The model under review builds one solid part; all positions refer to its coordinate system, in mm. Face numbers are marked on the shaded views. A direction names the side the tool comes from. Give positions to 0.01 mm unless a question says otherwise; leave off trailing zeros. Order: outer loops, then holes, each group sorted by start corner. A loop starts at its lowest first (then second) coordinate and runs counter-clockwise, first axis right, second up. Notation, with made-up numbers: (-3.75, 4) -> (50.25, 4) arc R22 cw to (50.25, 29) -> close; hole circle Ø9 at (63.5, 55). An arc over 180 degrees is marked (long way). Use one line per item in the form item = value.
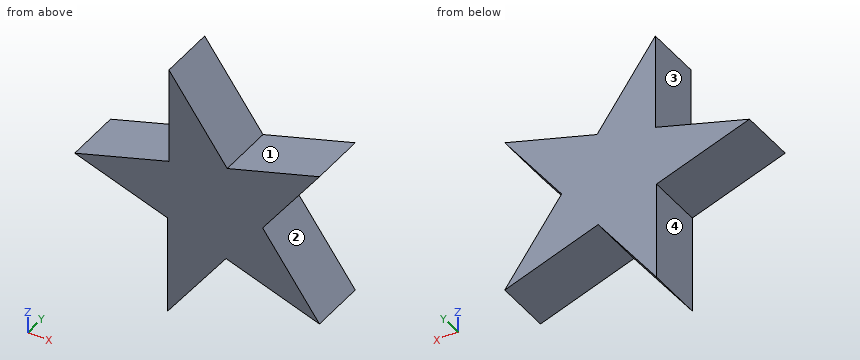
Autodesk Inventor part; units mm, degrees
ref_plane "YZ Plane" through (0, 0, 0) normal (1, 0, 0) x (0, 1, 0)
ref_plane "XZ Plane" through (0, 0, 0) normal (0, 1, 0) x (-1, 0, 0)
ref_plane "XY Plane" through (0, 0, 0) normal (0, 0, 1) x (1, 0, 0)
sketch "Эскиз1" plane through (0, 0, 0) normal (0, 1, 0) x (-1, 0, 0)
  circle A0 centre (141.9995, 431.0309) radius 94.7983
  line L0 (141.9995, 613.3951) -> (141.9995, 248.6146)
  line L1 (141.9995, 431.0309) -> (232.158, 401.7366)
  line L2 (170.6201, 521.4056) -> (170.6201, 453.1496)
  line L3 (171.4591, 340.9262) -> (171.4591, 410.4158)
  line L4 (171.4591, 340.9262) -> (130.4621, 397.3537)
  line L5 (64.7967, 486.044) -> (129.6246, 464.9802)
  line L6 (64.7967, 486.044) -> (104.7661, 431.0309)
  line L7 (170.6201, 453.1496) -> (236.7967, 431.4888)
  line L8 (236.7967, 431.4888) -> (171.4591, 410.4158)
  line L9 (130.4621, 397.3537) -> (64.7967, 376.0177)
  line L10 (64.7967, 376.0177) -> (104.7661, 431.0309)
  line L11 (170.6201, 521.4056) -> (129.6246, 464.9802)
  point P0 (141.9995, 431.0049)
  dimension "d22" = 172
  dimension "d24" = 172
  dimension "d27" = 72
  dimension "d41" = 36
  dimension "d43" = 36
  dimension "d44" = 36
  dimension "d45" = 36
  dimension "d46" = 36
extrude "Выдавливание1" add sketch "Эскиз1" against normal blind 39 contours L8 L1 L0 L11 L2 L7 | L8 L3 L4 L0 L1 | L0 L4 L9 L10 L6 L5 L11
1. Add section D-D on x = -186. Give the boundary of the cut face in (y, z).
Values:
outline = (-39, 415.11) -> (0, 415.11) -> (0, 448.12) -> (-39, 448.12) -> close
2. Add section A-A on x = -86.5. Give the boundary of the cut face in (y, z).
Values:
outline = (-39, 383.07) -> (0, 383.07) -> (0, 405.89) -> (-39, 405.89) -> close; (-39, 456.17) -> (0, 456.17) -> (0, 478.99) -> (-39, 478.99) -> close
3. Tool access review of the marked faces 1, 2, 3 and 4: name each direction out of +Z, -Z, +X, -X, +Y, -Y from which nothing blocks a thin tool from reaching the whole face with its end or side.
Values:
face_1 = +Z, +Y, -Y
face_2 = +X, +Y, -Y
face_3 = +Z, -X, +Y, -Y
face_4 = -Z, -X, +Y, -Y
4. For pin 1 Ø8 at (x, y) = (-133.5, -28.5) entering from -Z; pin 2 Ø1.5 at (x, y) = (-191, -13.5) entering from +Z; pin 3 Ø1.5 at (y, z) = (-4.5, 388.5) entering from +X; pin 4 Ø3 at (x, z) = (-97.5, 436.5) entering from +Y, all flat-tipped, find the tip position at first contact; note any pin that passes through.
Values:
pin_1 = 387.67
pin_2 = 446.72
pin_3 = -73.32
pin_4 = through
5. For L1, parallel to Z at x = -93, y = -30.5; L2, parallel to Z at x = -109.5, y = -8; L3, parallel to Z at x = -225, y = -3, list the stretches that pass through material, from the lowest coordinate up.
Values:
L1 = 385.18 to 414.84, 447.23 to 476.88
L2 = 390.54 to 471.52
L3 = 427.68 to 435.35
6. Add section C-C on y = -19. Give the boundary of the cut face in (x, z), then the cut area to 3 significant figures.
Values:
outline = (-236.8, 431.49) -> (-171.46, 410.42) -> (-171.46, 340.93) -> (-130.46, 397.35) -> (-64.8, 376.02) -> (-104.77, 431.03) -> (-64.8, 486.04) -> (-129.62, 464.98) -> (-170.62, 521.41) -> (-170.62, 453.15) -> close
area = 10,100 mm^2
7. Add section B-B on z = 383.5. Give the boundary of the cut face in (x, y), then the cut area to 3 significant figures.
Values:
outline = (-171.46, -39) -> (-140.53, -39) -> (-140.53, 0) -> (-171.46, 0) -> close; (-87.82, -39) -> (-70.23, -39) -> (-70.23, 0) -> (-87.82, 0) -> close
area = 1,890 mm^2
